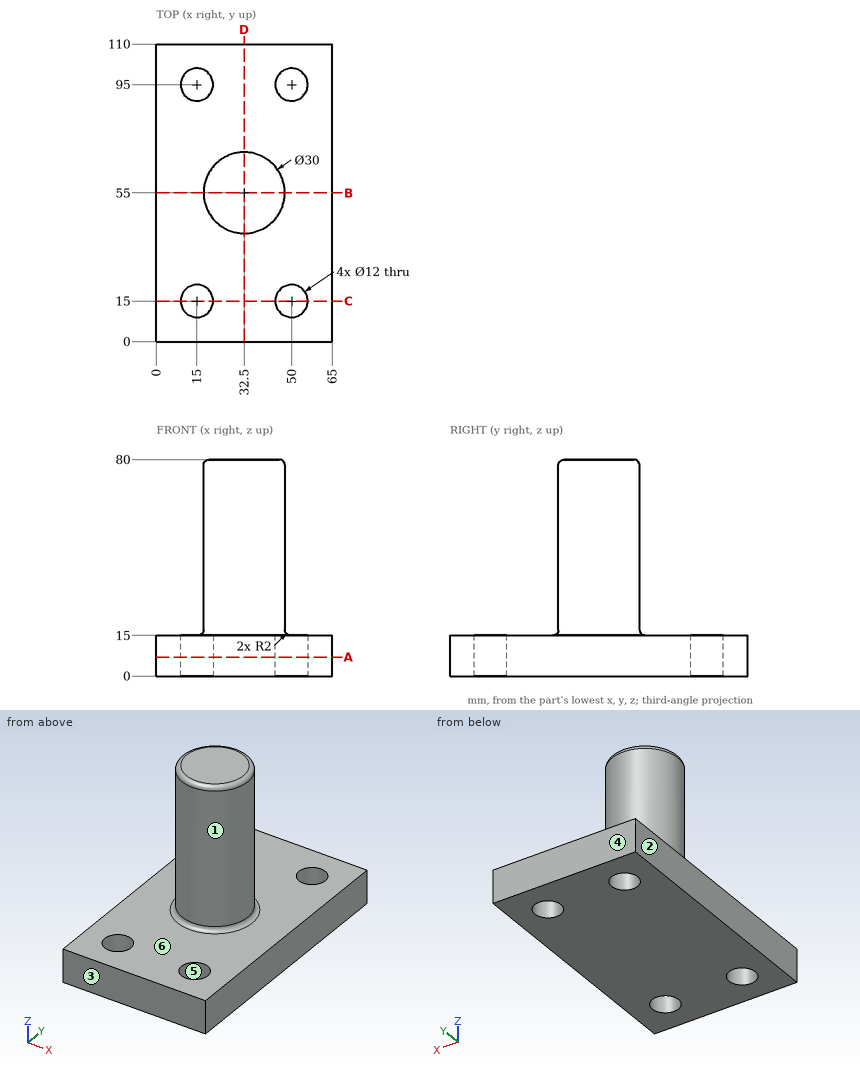
Source: three-view drawing plus pictorial views. Frame: mm from the lowest corner of the part. A direction names the side the tool comes from. Coordinates: 2 decimals unless noted, no trailing zeros. Order: outer loops, then holes, each group sorted by start corner. A loop starts at its lowest first (then second) coordinate and runs counter-clockwise, first axis right, second up.
1) Section B-B (y = 55). Return loops of the section in (x, z).
Result sheet:
outline: (0, 0) - (65, 0) - (65, 15) - (49.5, 15) arc R2 cw to (47.5, 17) - (47.5, 78) arc R2 ccw to (45.5, 80) - (19.5, 80) arc R2 ccw to (17.5, 78) - (17.5, 17) arc R2 cw to (15.5, 15) - (0, 15) - close
2) Set-up query: the marked faces 1 and 2. Return all of +Z, -Z, +X, -X, +Y, -Y with unobstructed straight access to the full face (end or side cutting, diameter ignored); none if empty.
Result sheet:
face 1: +Z
face 2: +Z, -Z, -X, +Y, -Y
3) Section A-A (z = 7). Return loops of the section in (x, y).
Result sheet:
outline: (0, 0) - (65, 0) - (65, 110) - (0, 110) - close; hole circle Ø12 at (15, 15); hole circle Ø12 at (15, 95); hole circle Ø12 at (50, 15); hole circle Ø12 at (50, 95)
4) Section C-C (y = 15). Return loops of the section in (x, z).
Result sheet:
outline: (0, 0) - (9, 0) - (9, 15) - (0, 15) - close; (21, 0) - (44, 0) - (44, 15) - (21, 15) - close; (56, 0) - (65, 0) - (65, 15) - (56, 15) - close
5) First-contact query: P1, Ø3, axis at y = 56.5, z = 51, coming from the +X side; P2, Ø12, axis at x = 48, y = 88, coming from the +Z side; P3, Ø7, axis at x = 15, y = 15, coming from the -Z side. Flat tips, straight axial feed; report the tip coordinate or a pass-through.
Result sheet:
P1: stops at x = 47.5
P2: stops at z = 15
P3: passes through
6) Ray query, probe 1 along Y at (x, z) = (15, 7.25); probe 2 along Z at (x, y) = (15, 31.5); probe 3 along Y at (x, z) = (52, 9). Return the intervals inside material, ascending.
Result sheet:
probe 1: y = 0 to 9, 21 to 89, 101 to 110
probe 2: z = 0 to 15
probe 3: y = 0 to 9.34, 20.66 to 89.34, 100.66 to 110
7) Section D-D (x = 32.5). Return loops of the section in (y, z).
Result sheet:
outline: (0, 0) - (110, 0) - (110, 15) - (72, 15) arc R2 cw to (70, 17) - (70, 78) arc R2 ccw to (68, 80) - (42, 80) arc R2 ccw to (40, 78) - (40, 17) arc R2 cw to (38, 15) - (0, 15) - close
8) Draft query along Y for the marked faces 3, 4, 5 and 6. Return one class per face: released by +Y, released by -Y, zero draft, split by the parting line, or undercut.
Result sheet:
face 3: released by -Y
face 4: released by +Y
face 5: undercut
face 6: zero draft
